Autodesk Inventor part; units mm, degrees
ref_plane "YZ Plane" through (0, 0, 0) normal (1, 0, 0) x (0, 1, 0)
ref_plane "XZ Plane" through (0, 0, 0) normal (0, 1, 0) x (-1, 0, 0)
ref_plane "XY Plane" through (0, 0, 0) normal (0, 0, 1) x (1, 0, 0)
sketch "Sketch1" plane through (0, 0, 0) normal (0, 1, 0) x (-1, 0, 0)
  circle A0 centre (0, 0) radius 25
  circle A1 centre (0, 0) radius 30
  circle A2 centre (0, 0) radius 17.5
  line L0 (0, 0) -> (25, 0) construction
  circle A3 centre (17.6777, -17.6777) radius 2
  circle A4 centre (17.6777, 17.6777) radius 2
  circle A5 centre (-17.6777, 17.6777) radius 2
  circle A6 centre (-17.6777, -17.6777) radius 2
  point P0 (0, -27.5)
  point P1 (0, -27.5)
  point P2 (27.5, 0)
  point P3 (-27.5, 0)
  point P4 (0, 27.5)
  dimension "d0" = 50
  dimension "d1" = 60
  dimension "d17" = 27.5
  dimension "d18" = 27.5
  dimension "d19" = 27.5
  dimension "d20" = 27.5
  dimension "d28" = 35
  dimension "d30" = 4
  dimension "d33" = 360
extrude "Extrusion1" add sketch "Sketch1" along normal blind 5 contours A0 A4 | A3 A0 | A0 A5 | A6 A0 | A1 picked at (18.1752, 18.1125) picked at (18.1752, -18.1125) picked at (-18.083, 18.1995) picked at (-18.083, -18.1995)
extrude "Extrusion2" add sketch "Sketch1" against normal blind 5 contours A0 A3 A6 A5 A4 | A4 A0 | A0 A4 | A3 A0 | A0 A3 | A5 A0 | A0 A5 | A6 A0 | A0 A6 | A1
hole "Hole2" at (0, 0, -27.5) at (-27.5, 0, 0) at (27.5, 0, 0) at (0, 0, 27.5) direction (0, 1, 0) diameter 2.45 end through all both
sketch "Sketch3" plane through (0, -5, 0) normal (0, -1, 0) x (1, 0, 0)
  circle A0 centre (16.0335, 14.9787) radius 3
  circle A1 centre (-15.7294, 16.8799) radius 3
  circle A2 centre (-17.6307, -14.8831) radius 3
  circle A3 centre (14.1323, -16.7843) radius 3
  point P0 (0, 0)
extrude "Extrusion4" cut sketch "Sketch3" against normal blind 10
properties part number "Placeholderjointouterring" material "Aluminum 6061-AHC"
Input: part model. Units: mm. Frame: model coordinates. A direction names the side the tool comes from. Round coordinates to 2 decimals unless told otherwise and drop trailing zeros. Loops run counter-clockwise (first coordinate to the right, second up) from the corner with the lowest first, then second, coordinate; pieces in that order, holes last. Notation, with made-up numbers: (-27, -4.75) -> (32, -4.75) arc R27 cw to (32, 11.25) -> close; hole circle Ø9 at (45, -35). An arc over 180 degrees is marked (long way). One line per item, written item: value.
(1) Material intervals for line 1 (Z direction, x = 0, y = -3.3) (3 decimals); line 2 (Z direction, x = 0, y = 2.55) (3 decimals); line 3 (X direction, y = -3.5, z = 13), sorted ascending. Write a range as [from, to].
Geometry check:
line 1: [-30, -28.725], [-26.275, -17.5], [17.5, 26.275], [28.725, 30]
line 2: [-30, -28.725], [-26.275, -25], [25, 26.275], [28.725, 30]
line 3: [-27.04, -11.72], [11.72, 13.78], [18.29, 27.04]
(2) Mould query, pull axis Z, two halves, no side actions, for faces 3 (the face through (18, 5, 18)), 4 (the face through (26.285, 0.07, 0.159)), 5 (the face through (29.97, -0.07, -1.32)), 6 (the face through (-0.368, 0.07, 26.332)). Classes: pulls with the +Z half, pulls with the -Z half, needs draft (parallel to the pull), parting line crosses it, or undercut.
Geometry check:
face 3: needs draft
face 4: undercut
face 5: parting line crosses it
face 6: undercut
(3) Section B-B (x = 0). Return the cut outline in (y, z) (3 decimals), plus the area to 3 significant figures.
Geometry check:
outline: (-5, -30) -> (5, -30) -> (5, -28.725) -> (-5, -28.725) -> close; (-5, -26.275) -> (5, -26.275) -> (5, -25) -> (0, -25) -> (0, -17.5) -> (-5, -17.5) -> close; (-5, 17.5) -> (0, 17.5) -> (0, 25) -> (5, 25) -> (5, 26.275) -> (-5, 26.275) -> close; (-5, 28.725) -> (5, 28.725) -> (5, 30) -> (-5, 30) -> close
area: 126 mm2
(4) Set-up query: faces 1 (the face through (-24.94, 2.46, 1.73)), 2 (the face through (-0.368, 0.07, -28.668)). Return all of +Z, -Z, +X, -X, +Y, -Y with unobstructed straight access to the full face (end or side cutting, diameter ignored); none if empty.
Geometry check:
face 1: +Y
face 2: +Y, -Y
(5) Section C-C (y = 2.25). Return the cut outline in (x, z) (3 decimals).
Geometry check:
outline: circle Ø60 at (0, 0); hole circle Ø2.45 at (-27.5, 0); hole (-20.558, -14.226) arc R3 ccw to (-17.474, -17.879) arc R25 ccw (long way) to (-15.217, 19.836) arc R3 ccw to (-18.714, 16.577) arc R25 ccw to start; hole circle Ø2.45 at (0, -27.5); hole circle Ø2.45 at (0, 27.5); hole circle Ø2.45 at (27.5, 0)
(6) Section A-A (z = 0). Return the cut outline in (x, y) (3 decimals), plus the area to 3 significant figures.
Geometry check:
outline: (-30, -5) -> (-28.725, -5) -> (-28.725, 5) -> (-30, 5) -> close; (-26.275, -5) -> (-17.5, -5) -> (-17.5, 0) -> (-25, 0) -> (-25, 5) -> (-26.275, 5) -> close; (17.5, -5) -> (26.275, -5) -> (26.275, 5) -> (25, 5) -> (25, 0) -> (17.5, 0) -> close; (28.725, -5) -> (30, -5) -> (30, 5) -> (28.725, 5) -> close
area: 126 mm2
(7) Pin query (flat end, axial travel): pin 1 (8 mm diameter, centred on x = -15.73, z = 16.88, fed in from +Y); pin 2 (5 mm diameter, centred on x = 16.03, z = 14.98, fed in from -Y); pin 3 (3 mm diameter, centred on y = 1.5, z = -20.5, fed in from +X); pin 4 (2 mm diameter, centred on x = -7, y = 2, fed in from -Z). Return the tip coordinate at first contact, or that it passes through.
Geometry check:
pin 1: y = 5
pin 2: through
pin 3: x = 23.22
pin 4: z = -29.39
(8) Section D-D (z = 10). Return the cut outline in (x, y), plus the area to 3 significant figures.
Geometry check:
outline: (-28.28, -5) -> (-14.36, -5) -> (-14.36, 0) -> (-22.91, 0) -> (-22.91, 5) -> (-28.28, 5) -> close; (14.36, -5) -> (28.28, -5) -> (28.28, 5) -> (22.91, 5) -> (22.91, 0) -> (14.36, 0) -> close
area: 193 mm2
